from build123d import *

# Parameters (mm, degrees)
F0_W     = 78
F0_H     = 53.5
F1_DEPTH = 2.4
F2_DEPTH = 6
F3_W     = 66
F3_H     = 41.5
F4_DEPTH = 3.5
F5_SIZE  = 1


with BuildPart() as f1:
    # F0 (on Top) → F1 (new body)
    with BuildSketch(Plane.XY):
        with Locations((24.061151, -25.793475)):
            Rectangle(F0_W, F0_H)
        with BuildLine():
            Line((-10.938849, -8.77954), (-10.938849, -3.043475))
            Line((-10.938849, -3.043475), (-6.991661, -3.043475))
            ThreePointArc((-6.991661, -3.043475), (-6.173105, -2.505917), (-5.354548, -3.043475))
            Line((-5.354548, -3.043475), (22.380689, -3.043475))
            ThreePointArc((22.380689, -3.043475), (23.22092, -2.450647), (24.061151, -3.043475))
            Line((24.061151, -3.043475), (55.158719, -3.043475))
            ThreePointArc((55.158719, -3.043475), (55.675749, -2.828865), (56.192778, -3.043475))
            Line((56.192778, -3.043475), (59.061151, -3.043475))
            Line((59.061151, -3.043475), (59.061151, -8.429402))
            ThreePointArc((59.061151, -8.429402), (59.415671, -9.148699), (59.061151, -9.867996))
            Line((59.061151, -9.867996), (59.061151, -38.373694))
            ThreePointArc((59.061151, -38.373694), (59.364159, -38.895946), (59.061151, -39.418198))
            Line((59.061151, -39.418198), (59.061151, -48.543475))
            Line((59.061151, -48.543475), (54.673515, -48.543475))
            ThreePointArc((54.673515, -48.543475), (52.858135, -49.124567), (51.042754, -48.543475))
            Line((51.042754, -48.543475), (26.816798, -48.543475))
            ThreePointArc((26.816798, -48.543475), (25.438975, -49.262858), (24.061151, -48.543475))
            Line((24.061151, -48.543475), (-1.533683, -48.543475))
            ThreePointArc((-1.533683, -48.543475), (-3.096999, -49.304078), (-4.660315, -48.543475))
            Line((-4.660315, -48.543475), (-10.938849, -48.543475))
            Line((-10.938849, -48.543475), (-10.938849, -41.287743))
            ThreePointArc((-10.938849, -41.287743), (-11.387766, -39.830718), (-10.938849, -38.373694))
            Line((-10.938849, -38.373694), (-10.938849, -11.72171))
            ThreePointArc((-10.938849, -11.72171), (-11.712319, -10.250625), (-10.938849, -8.77954))
        make_face(mode=Mode.SUBTRACT)
    extrude(amount=F1_DEPTH)

    # F0 (on Top) → F2 (join)
    with BuildSketch(Plane.XY):
        with BuildLine():
            Line((-6.991661, -3.043475), (-10.938849, -3.043475))
            Line((-10.938849, -3.043475), (-10.938849, -8.77954))
            ThreePointArc((-10.938849, -8.77954), (-11.712319, -10.250625), (-10.938849, -11.72171))
            Line((-10.938849, -11.72171), (-10.938849, -38.373694))
            ThreePointArc((-10.938849, -38.373694), (-11.387766, -39.830718), (-10.938849, -41.287743))
            Line((-10.938849, -41.287743), (-10.938849, -48.543475))
            Line((-10.938849, -48.543475), (-4.660315, -48.543475))
            ThreePointArc((-4.660315, -48.543475), (-3.096999, -49.304078), (-1.533683, -48.543475))
            Line((-1.533683, -48.543475), (24.061151, -48.543475))
            ThreePointArc((24.061151, -48.543475), (25.438975, -49.262858), (26.816798, -48.543475))
            Line((26.816798, -48.543475), (51.042754, -48.543475))
            ThreePointArc((51.042754, -48.543475), (52.858135, -49.124567), (54.673515, -48.543475))
            Line((54.673515, -48.543475), (59.061151, -48.543475))
            Line((59.061151, -48.543475), (59.061151, -39.418198))
            ThreePointArc((59.061151, -39.418198), (59.364159, -38.895946), (59.061151, -38.373694))
            Line((59.061151, -38.373694), (59.061151, -9.867996))
            ThreePointArc((59.061151, -9.867996), (59.415671, -9.148699), (59.061151, -8.429402))
            Line((59.061151, -8.429402), (59.061151, -3.043475))
            Line((59.061151, -3.043475), (56.192778, -3.043475))
            ThreePointArc((56.192778, -3.043475), (55.675749, -2.828865), (55.158719, -3.043475))
            Line((55.158719, -3.043475), (24.061151, -3.043475))
            ThreePointArc((24.061151, -3.043475), (23.22092, -2.450647), (22.380689, -3.043475))
            Line((22.380689, -3.043475), (-5.354548, -3.043475))
            ThreePointArc((-5.354548, -3.043475), (-6.173105, -2.505917), (-6.991661, -3.043475))
        make_face()
    extrude(amount=F2_DEPTH)

    # F3 (on face) → F4 (cut)
    with BuildSketch(Plane.XY.offset(6)):
        with Locations((24.061151, -25.793475)):
            Rectangle(F3_W, F3_H)
    extrude(amount=-F4_DEPTH, mode=Mode.SUBTRACT)

    # F5
    f5_edges = [f1.edges().sort_by_distance(p)[0] for p in [
        (-8.938849, -25.793475, 2.5),
        (24.061151, -5.043475, 2.5),
        (57.061151, -25.793475, 2.5),
        (24.061151, -46.543475, 2.5),
    ]]
    chamfer(f5_edges, length=F5_SIZE)


solid = f1.part
The listing builds one solid part. Answer for the finished solid, in the listing's coordinates (mm). A direction names the side the tool comes from. Round coordinates to 2 decimals unless told otherwise and drop trailing zeros. Order: outer loops, then holes, each group sorted by start corner. A loop starts at its lowest first (then second) coordinate and runs counter-clockwise, first axis right, second up. Notation, with made-up numbers: (-19, 87) -> (-10, 87) arc R22 cw to (-10, 114) -> close; hole circle Ø5 at (-30, 49.25). An arc over 180 degrees is marked (long way). Write each question's results on one line, items separated by ' | '. Start each with the question number.
Q1. Each of these flat-tipped pins is pushed along its axis until it touches: pin 1 (1 mm diameter, centred on x = 25.5, y = -33, fed in from -Z); pin 2 (1.1 mm diameter, centred on x = -10, z = 4.5, fed in from +Y); pin 3 (1.1 mm diameter, centred on x = -8, z = 3.5, fed in from -Y); pin 4 (1.8 mm diameter, centred on y = -43, z = 4, fed in from +X). Where does it stop, or does it pass through?
Q2. Straight lines are drawn through the part: probe 1 along X at (y, z) = (-37, 4.8); probe 2 along Y at (x, z) = (46, 4.8); probe 3 along Y at (x, z) = (23.5, 4). For each, find the intervals that lie inside material, in ascending order. Write a range as from..to.
Q3. Which of the six approach directions +Z, -Z, +X, -X, +Y, -Y give full straight-line access (tool end or side, diameter ignored) to faces 1 (the flat face through (-10.939, -6, 4)), 2 (the cylindrical face through (-6.159, -2.506, 4.175)), 3 (the flat face through (24, -26, 2.5)), 4 (the flat face through (59.061, -24, 4))?
Q4. The mould has two halves that part along Y. Classify faces 5 (the cylindrical face through (59.416, -9.16, 4.175)), 6 (the flat face through (-8, -48.543, 4)), 7 (the flat face through (21, -47, 6)): pulls with the +Y half, pulls with the -Y half, needs draft (parallel to the pull), parting line crosses it, or undercut.
Q5. Find section A-A (z = 4.7). Determine the outline of the cut face in (x, y).
Q6. Find section D-D (x = 12). Determine the outline of the cut face in (y, z).
Q7. Find section B-B (x = -10). Determine the outline of the cut face in (y, z), then the cut area to 3 significant figures.
Q8. Find section C-C (y = -47.5). Determine the outline of the cut face in (x, z), then the cut area to 3 significant figures.
Worked answers:
1) pin 1: stops at z = 0 | pin 2: stops at y = -3.04 | pin 3: stops at y = -48.54 | pin 4: stops at x = 59.06
2) probe 1: x = -10.94..-8.94, 57.06..59.06 | probe 2: y = -48.54..-46.54, -5.04..-3.04 | probe 3: y = -48.54..-46.54, -5.04..-2.5
3) face 1: +Z, -X, +Y | face 2: +Z, +Y | face 3: +Z | face 4: +Z, +X
4) face 5: undercut | face 6: pulls with the -Y half | face 7: needs draft
5) outline: (-10.94, -48.54) -> (-4.66, -48.54) arc R1.99 ccw to (-1.53, -48.54) -> (24.06, -48.54) arc R1.68 ccw to (26.82, -48.54) -> (51.04, -48.54) arc R3.13 ccw to (54.67, -48.54) -> (59.06, -48.54) -> (59.06, -39.42) arc R0.6 ccw to (59.06, -38.37) -> (59.06, -9.87) arc R0.91 ccw to (59.06, -8.43) -> (59.06, -3.04) -> (56.19, -3.04) arc R0.73 ccw to (55.16, -3.04) -> (24.06, -3.04) arc R0.89 ccw to (22.38, -3.04) -> (-5.35, -3.04) arc R0.89 ccw to (-6.99, -3.04) -> (-10.94, -3.04) -> (-10.94, -8.78) arc R1.79 ccw to (-10.94, -11.72) -> (-10.94, -38.37) arc R2.59 ccw to (-10.94, -41.29) -> close; hole (-8.94, -46.54) -> (57.06, -46.54) -> (57.06, -5.04) -> (-8.94, -5.04) -> close
6) outline: (-52.54, 0) -> (0.96, 0) -> (0.96, 2.4) -> (-3.04, 2.4) -> (-3.04, 6) -> (-5.04, 6) -> (-5.04, 3.5) -> (-6.04, 2.5) -> (-45.54, 2.5) -> (-46.54, 3.5) -> (-46.54, 6) -> (-48.54, 6) -> (-48.54, 2.4) -> (-52.54, 2.4) -> close
7) outline: (-52.54, 0) -> (0.96, 0) -> (0.96, 2.4) -> (-3.04, 2.4) -> (-3.04, 6) -> (-48.54, 6) -> (-48.54, 2.4) -> (-52.54, 2.4) -> close | area: 292 mm2
8) outline: (-14.94, 0) -> (63.06, 0) -> (63.06, 2.4) -> (59.06, 2.4) -> (59.06, 6) -> (-10.94, 6) -> (-10.94, 2.4) -> (-14.94, 2.4) -> close | area: 439 mm2
